The listing builds one solid part. Answer for the finished solid, in the listing's coordinates (mm). Face numbers are marked on the shaded views. A direction names the side the tool comes from. Coordinates: 2 decimals unless noted, no trailing zeros. Order: outer loops, then holes, each group sorted by start corner. A loop starts at its lowest first (then second) coordinate and runs counter-clockwise, first axis right, second up. Notation, with made-up numbers: (35.5, 1) - (50.5, 1) arc R32 ccw to (50.5, 32) - close; hole circle Ø5 at (-23, 31.25). An arc over 180 degrees is marked (long way). Use a Markdown table: item, result. Add a question column.
Item 1: The part is cut by section C-C, the plane x = -160.5. Give the vertices of the cut face in (y, z).
Item 2: The part is cut by section B-B, the plane z = 358. Give the vertices of the cut face in (x, y), then the cut area to 3 significant figures.
Item 3: The part is cut by section D-D, the plane y = -98.5. Give the vertices of the cut face in (x, z).
Item 4: The mould has two halves that part along Z. Classify the marked faces 1, 2 and 3: released by +Z, released by -Z, zero draft, split by the parting line, or undercut.
Item 5: Flat-ended cylindrical pins translate along their axes: P1, Ø5, axis at x = -4.5, y = -48.5, coming from the +Z side; P2, Ø1.5, axis at y = -145.5, z = 104.5, coming from the -X side; P3, Ø21, axis at y = -138, z = 417, coming from the +X side. Find the tip coordinate at first contact, or state that the pin passes through.
Item 6: Find the intervals of material crossed by line 1 along X through (y, z) = (-34, 579); line 2 along Z through (x, y) = (-223.5, -18.5); line 3 along Y through (x, z) = (-271.5, 647), in increasing order.
Item 7: The part is cut by section A-A, the plane y = -166. Give the vertices of the cut face in (x, z), then the cut area to 3 significant figures.
Item 8: For the marked faces 4, 5, 6 and 7, determine the directions among +Z, -Z, +X, -X, +Y, -Y from which every point of the face is accessible in a straight line to the end or side of a thin tool.
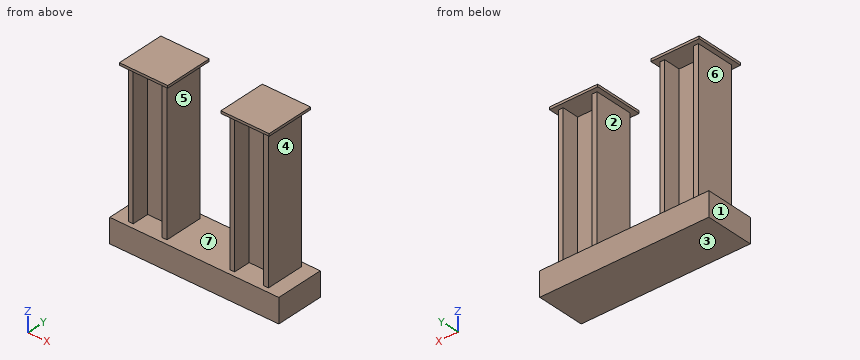
from build123d import *

# Parameters (mm, degrees)
F0_W     = 350
F0_H     = 100
F1_DEPTH = 200
F3_DEPTH = 600
F4_W     = 200
F4_H     = 200
F5_DEPTH = 10


with BuildPart() as f1:
    # F0 (on Front) → F1 (new body)
    with BuildSketch(Plane.XZ):
        with Locations((-175, 50)):
            Rectangle(F0_W, F0_H)
        with Locations((175, 50)):
            Rectangle(F0_W, F0_H)
    extrude(amount=F1_DEPTH)

    # F2 (on face) → F3 (join)
    with BuildSketch(Plane.XY.offset(100)):
        Polygon((-130, -180), (-130, -20), (-150, -20), (-150, -90), (-270, -90), (-270, -20), (-290, -20), (-290, -180), (-270, -180), (-270, -110), (-150, -110), (-150, -180), align=None)
        Polygon((150, -20), (130, -20), (130, -180), (150, -180), (150, -110), (270, -110), (270, -180), (290, -180), (290, -20), (270, -20), (270, -90), (150, -90), align=None)
    extrude(amount=F3_DEPTH)

    # F4 (on face) → F5 (join)
    with BuildSketch(Plane.XY.offset(700)):
        with Locations((210, -100)):
            Rectangle(F4_W, F4_H)
        Polygon((130, -20), (150, -20), (150, -90), (270, -90), (270, -20), (290, -20), (290, -180), (270, -180), (270, -110), (150, -110), (150, -180), (130, -180), align=None, mode=Mode.SUBTRACT)
        Polygon((150, -90), (150, -20), (130, -20), (130, -180), (150, -180), (150, -110), (270, -110), (270, -180), (290, -180), (290, -20), (270, -20), (270, -90), align=None)
        with Locations((-210, -100)):
            Rectangle(F4_W, F4_H)
    extrude(amount=-F5_DEPTH)


solid = f1.part
Solution:
| question | item | result |
|---|---|---|
| 1 | outline | (-200, 0) - (0, 0) - (0, 100) - (-90, 100) - (-90, 690) - (0, 690) - (0, 700) - (-200, 700) - (-200, 690) - (-110, 690) - (-110, 100) - (-200, 100) - close |
| 2 | outline | (-290, -180) - (-270, -180) - (-270, -110) - (-150, -110) - (-150, -180) - (-130, -180) - (-130, -20) - (-150, -20) - (-150, -90) - (-270, -90) - (-270, -20) - (-290, -20) - close; (130, -180) - (150, -180) - (150, -110) - (270, -110) - (270, -180) - (290, -180) - (290, -20) - (270, -20) - (270, -90) - (150, -90) - (150, -20) - (130, -20) - close |
| 2 | area | 17,600 mm2 |
| 3 | outline | (-350, 0) - (350, 0) - (350, 100) - (290, 100) - (290, 690) - (310, 690) - (310, 700) - (110, 700) - (110, 690) - (130, 690) - (130, 100) - (-130, 100) - (-130, 690) - (-110, 690) - (-110, 700) - (-310, 700) - (-310, 690) - (-290, 690) - (-290, 100) - (-350, 100) - close |
| 4 | face 1 | zero draft |
| 4 | face 2 | undercut |
| 4 | face 3 | released by -Z |
| 5 | P1 | stops at z = 100 |
| 5 | P2 | stops at x = -290 |
| 5 | P3 | stops at x = 290 |
| 6 | line 1 | x = -290 to -270, -150 to -130, 130 to 150, 270 to 290 |
| 6 | line 2 | z = 0 to 100, 690 to 700 |
| 6 | line 3 | y = -180 to -20 |
| 7 | outline | (-350, 0) - (350, 0) - (350, 100) - (290, 100) - (290, 690) - (310, 690) - (310, 700) - (110, 700) - (110, 690) - (130, 690) - (130, 100) - (-130, 100) - (-130, 690) - (-110, 690) - (-110, 700) - (-310, 700) - (-310, 690) - (-290, 690) - (-290, 100) - (-350, 100) - close; hole (-270, 100) - (-150, 100) - (-150, 690) - (-270, 690) - close; hole (150, 100) - (270, 100) - (270, 690) - (150, 690) - close |
| 7 | area | 121,000 mm2 |
| 8 | face 4 | +X, +Y, -Y |
| 8 | face 5 | +Y, -Y |
| 8 | face 6 | -X, +Y, -Y |
| 8 | face 7 | none |
